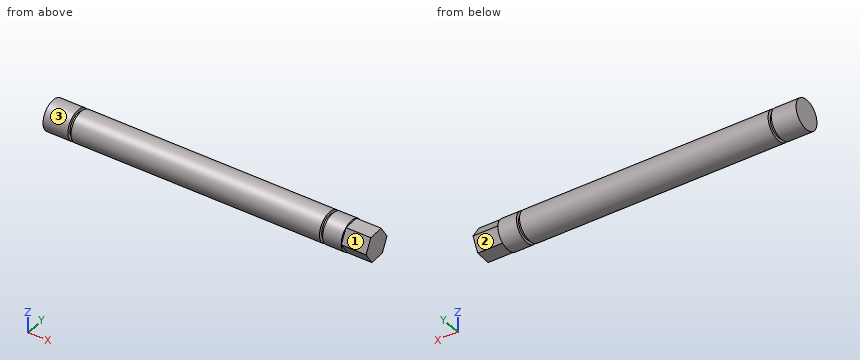
```python
from build123d import *

# Parameters (mm, degrees)
SKETCH2_R           = 7.62
BOSS_EXTRUDE1_DEPTH = 165.1
SKETCH3_W           = 1.6002
SKETCH3_H           = 1.6002
SKETCH4_R           = 7.62
SKETCH4_R_2         = 6.0198
CUT_EXTRUDE1_DEPTH  = 1.6002
SKETCH5_OUTSIDE_W   = 50.54
SKETCH5_OUTSIDE_H   = 50.54
CUT_EXTRUDE2_DEPTH  = 12.7


with BuildPart() as part:
    # Sketch2 → Boss-Extrude1 (new body)
    with BuildSketch(Plane(origin=(0, 0, 0), x_dir=(0, 0, -1), z_dir=(1, 0, 0))):
        Circle(SKETCH2_R)
    extrude(amount=BOSS_EXTRUDE1_DEPTH)

    # Sketch3 → Cut-Revolve1 (revolve, cut)
    with BuildSketch(Plane.XY, mode=Mode.PRIVATE) as cut_revolve1_sk:
        with Locations((13.5001, 6.8199)):
            Rectangle(SKETCH3_W, SKETCH3_H)
    revolve(cut_revolve1_sk.sketch.rotate(Axis((0, 0, 0), (1, 0, 0)), 90), axis=Axis((0, 0, 0), (1, 0, 0)), mode=Mode.SUBTRACT)

    # Sketch4 → Cut-Extrude1 (cut)
    with BuildSketch(Plane.ZY.offset(-141.3002)):
        Circle(SKETCH4_R)
        Circle(SKETCH4_R_2, mode=Mode.SUBTRACT)
    extrude(amount=-CUT_EXTRUDE1_DEPTH, mode=Mode.SUBTRACT)

    # Sketch5 outside → Cut-Extrude2 (cut)
    with BuildSketch(Plane(origin=(165.1, 0, 0), x_dir=(0, 0, -1), z_dir=(1, 0, 0))):
        Rectangle(SKETCH5_OUTSIDE_W, SKETCH5_OUTSIDE_H)
        Polygon((6.366186157, 4.187609558), (-0.44348318, 7.607083716), (-6.809669337, 3.419474158), (-6.366186157, -4.187609558), (0.44348318, -7.607083716), (6.809669337, -3.419474158), align=None, mode=Mode.SUBTRACT)
    extrude(amount=-CUT_EXTRUDE2_DEPTH, mode=Mode.SUBTRACT)


solid = part.part
```
Source: CAD feature listing. Evaluate the final solid. Frame: model axes, mm. Face numbers are marked on the shaded views. A direction names the side the tool comes from. Round coordinates to 2 decimals unless told otherwise and drop trailing zeros. Order: outer loops, then holes, each group sorted by start corner. A loop starts at its lowest first (then second) coordinate and runs counter-clockwise, first axis right, second up. Notation, with made-up numbers: (-1, 84.5) -> (24, 84.5) arc R26 ccw to (24, 121.5) -> close; hole circle Ø2 at (74.25, 38). An arc over 180 degrees is marked (long way). One line per item, written item: value. Start each with the question number.
Q1. Section query B-B (y = -1.5). Return the cut outline in (x, z).
Q2. Section query A-A (z = -3.25). Return the cut outline in (x, y), plus the area to 3 significant figures.
Q3. Section query C-C (x = 51). Return the cut outline in (y, z), plus the area to 3 significant figures.
Q4. Material intervals for probe 1 along X at (y, z) = (2, -6); probe 2 along X at (y, z) = (4, 6.25); probe 3 along Y at (x, z) = (51, 0.75), sorted ascending.
Q5. Access query for the marked faces 1, 2 and 3. Directions: +Z, -Z, +X, -X, +Y, -Y. A direction counts if a zero-diameter tool reaches every point of the face in a straight line with its end or side. Return the directions, or none.
Q6. Pin query (flat end, axial travel): pin 1 (3 mm diameter, centred on x = 133, z = 6, fed in from +Y); pin 2 (4 mm diameter, centred on x = 90, y = 1, fed in from -Z); pin 3 (1 mm diameter, centred on x = 41, z = 5.5, fed in from -Y); pin 4 (2 mm diameter, centred on x = 127, y = 3.5, fed in from -Z). Return the tip coordinate at first contact, or that it passes through.
Findings below:
1. outline: (0, -7.47) -> (12.7, -7.47) -> (12.7, -5.83) -> (14.3, -5.83) -> (14.3, -7.47) -> (141.3, -7.47) -> (141.3, -5.83) -> (142.9, -5.83) -> (142.9, -7.47) -> (152.4, -7.47) -> (152.4, -6.7) -> (165.1, -6.7) -> (165.1, 6.52) -> (152.4, 6.52) -> (152.4, 7.47) -> (142.9, 7.47) -> (142.9, 5.83) -> (141.3, 5.83) -> (141.3, 7.47) -> (14.3, 7.47) -> (14.3, 5.83) -> (12.7, 5.83) -> (12.7, 7.47) -> (0, 7.47) -> close
2. outline: (0, -6.89) -> (12.7, -6.89) -> (12.7, -5.07) -> (14.3, -5.07) -> (14.3, -6.89) -> (141.3, -6.89) -> (141.3, -5.07) -> (142.9, -5.07) -> (142.9, -6.89) -> (152.4, -6.89) -> (152.4, -5.76) -> (165.1, -5.76) -> (165.1, 5.75) -> (152.4, 5.75) -> (152.4, 6.89) -> (142.9, 6.89) -> (142.9, 5.07) -> (141.3, 5.07) -> (141.3, 6.89) -> (14.3, 6.89) -> (14.3, 5.07) -> (12.7, 5.07) -> (12.7, 6.89) -> (0, 6.89) -> close
2. area: 2,240 mm²
3. outline: circle Ø15.24 at (0, 0)
3. area: 182 mm²
4. probe 1: 0 to 12.7, 14.3 to 141.3, 142.9 to 165.1
4. probe 2: 0 to 12.7, 14.3 to 141.3, 142.9 to 152.4
4. probe 3: -7.58 to 7.58
5. face 1: +Z, +X, -Y
5. face 2: -Z, +X, +Y
5. face 3: +X, -X
6. pin 1: y = 6.15
6. pin 2: z = -7.62
6. pin 3: y = -5.75
6. pin 4: z = -7.2
